from build123d import *

# Parameters (mm, degrees)
F0_W     = 25.4
F0_H     = 25.4
F1_DEPTH = 736.6
F2_W     = 22.2504
F2_H     = 22.2504
F3_DEPTH = 736.6
F4_R     = 1.524
F5_R     = 0.254
F6_DEPTH = 226.9998


with BuildPart() as f1:
    # F0 (on Front) → F1 (new body)
    with BuildSketch(Plane.XZ):
        Rectangle(F0_W, F0_H)
    extrude(amount=F1_DEPTH)

    # F2 (on face) → F3 (cut, through all)
    with BuildSketch(Plane.XZ.offset(736.6)):
        Rectangle(F2_W, F2_H)
    extrude(amount=-F3_DEPTH, mode=Mode.SUBTRACT)

    # F4
    f4_edges = [f1.edges().sort_by_distance(p)[0] for p in [
        (-11.1252, -368.3, 11.1252),
        (11.1252, -368.3, -11.1252),
        (11.1252, -368.3, 11.1252),
        (-11.1252, -368.3, -11.1252),
    ]]
    fillet(f4_edges, radius=F4_R)

    # F5
    f5_edges = [f1.edges().sort_by_distance(p)[0] for p in [
        (12.7, -368.3, 12.7),
        (12.7, -368.3, -12.7),
        (-12.7, -368.3, -12.7),
        (-12.7, -368.3, 12.7),
    ]]
    fillet(f5_edges, radius=F5_R)

    # F6 (cut): a face of the model
    f6_faces = [f1.faces().sort_by_distance(p)[0] for p in [
        (12.3407897552, -736.6, 0),
    ]]
    extrude(f6_faces, amount=-F6_DEPTH, mode=Mode.SUBTRACT)


solid = f1.part
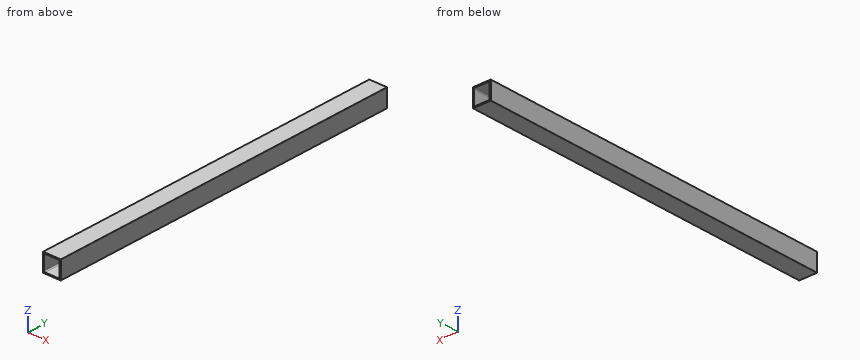
Model file for the job. Use its own axes, mm. Give positions to 0.01 mm unless a question says otherwise; leave off trailing zeros. Loops run counter-clockwise (first coordinate to the right, second up) from the corner with the lowest first, then second, coordinate; pieces in that order, holes last.
1) Saw through at A-A (y = -226.5). Write the cut outline in (x, z).
2) Wall check: line 1 (X direction, y = -252, z = 8.75); line 2 (X direction, y = -230, z = -10.25). Give the ranges that are in metal, low to high.
3) Saw through at B-B (z = -1.75). Write the cut outline in (x, y), plus the area to 3 significant figures.
4) Saw through at C-C (x = -5). Write the cut outline in (y, z).
Answer block:
1. outline: (-12.7, -12.45) arc R0.25 ccw to (-12.45, -12.7) - (12.45, -12.7) arc R0.25 ccw to (12.7, -12.45) - (12.7, 12.45) arc R0.25 ccw to (12.45, 12.7) - (-12.45, 12.7) arc R0.25 ccw to (-12.7, 12.45) - close; hole (-11.13, -9.6) arc R1.52 ccw to (-9.6, -11.13) - (9.6, -11.13) arc R1.52 ccw to (11.13, -9.6) - (11.13, 9.6) arc R1.52 ccw to (9.6, 11.13) - (-9.6, 11.13) arc R1.52 ccw to (-11.13, 9.6) - close
2. line 1: x = -12.7 to -11.13, 11.13 to 12.7
2. line 2: x = -12.7 to -10.98, 10.98 to 12.7
3. outline: (-12.7, -509.6) - (-11.13, -509.6) - (-11.13, 0) - (-12.7, 0) - close; (11.13, -509.6) - (12.7, -509.6) - (12.7, 0) - (11.13, 0) - close
3. area: 1,610 mm2
4. outline: (-509.6, -12.7) - (0, -12.7) - (0, -11.13) - (-509.6, -11.13) - close; (-509.6, 11.13) - (0, 11.13) - (0, 12.7) - (-509.6, 12.7) - close
